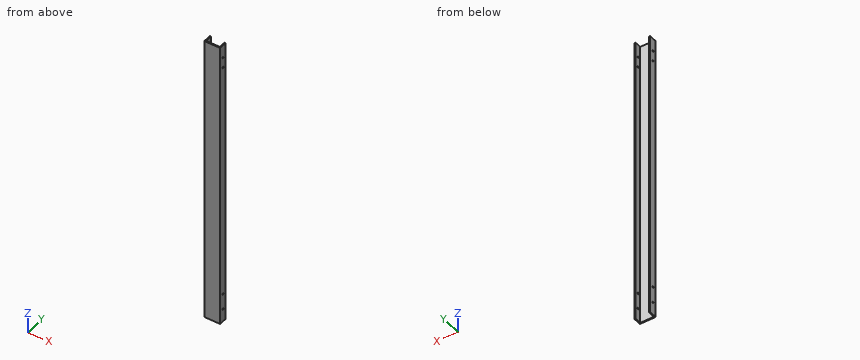
from build123d import *

# Parameters (mm, degrees)
EXTRUDE_1_DEPTH = 560.3
M4X0_7_1_D      = 3.3
M4X0_7_1_DEPTH  = 11.5
M4X0_7_1_TIP    = 0.991420021
M4X0_7_2_D      = 3.3
M4X0_7_2_DEPTH  = 11.5
M4X0_7_2_TIP    = 0.991420021
M4X0_7_4_D      = 3.3
M4X0_7_4_DEPTH  = 11.5
M4X0_7_4_TIP    = 0.991420021


with BuildPart() as part:
    # ｽｹｯﾁ1 → ﾎﾞｽ - 押し出し1 (new body)
    with BuildSketch(Plane.XY):
        Polygon((0, 0), (15, 0), (15, 15), (13, 15), (13, 2), (-13, 2), (-13, 15), (-15, 15), (-15, 0), align=None)
    extrude(amount=EXTRUDE_1_DEPTH)

    # M4x0.7 ねじ穴1
    with Locations(Plane(origin=(15, 7.5, 56), x_dir=(0, 0, 1), z_dir=(1, 0, 0))):
        with Locations((0, 0), (-31, 0)):
            Hole(M4X0_7_1_D / 2, depth=M4X0_7_1_DEPTH)
            with Locations((0, 0, -(M4X0_7_1_DEPTH + M4X0_7_1_TIP / 2))):  # 118° drill point
                Cone(0, M4X0_7_1_D / 2, M4X0_7_1_TIP, mode=Mode.SUBTRACT)

    # M4x0.7 ねじ穴2
    with Locations(Plane(origin=(15, 7.5, 535.3), x_dir=(0, 0, 1), z_dir=(1, 0, 0))):
        with Locations((0, 0), (-20, 0)):
            Hole(M4X0_7_2_D / 2, depth=M4X0_7_2_DEPTH)
            with Locations((0, 0, -(M4X0_7_2_DEPTH + M4X0_7_2_TIP / 2))):  # 118° drill point
                Cone(0, M4X0_7_2_D / 2, M4X0_7_2_TIP, mode=Mode.SUBTRACT)

    # M4x0.7 ねじ穴4
    with Locations(Plane(origin=(-15, 7.5, 56), x_dir=(0, 0, -1), z_dir=(-1, 0, 0))):
        with Locations((0, 0), (31, 0), (-459.3, 0), (-479.3, 0)):
            Hole(M4X0_7_4_D / 2, depth=M4X0_7_4_DEPTH)
            with Locations((0, 0, -(M4X0_7_4_DEPTH + M4X0_7_4_TIP / 2))):  # 118° drill point
                Cone(0, M4X0_7_4_D / 2, M4X0_7_4_TIP, mode=Mode.SUBTRACT)


solid = part.part
Check sheet for the modelled part. Datum: model origin and axes. Units: mm. Give positions to 0.01 mm unless a question says otherwise; leave off trailing zeros. Write each loop counter-clockwise with the first axis right and the second up, starting at its lowest first coordinate (ties: lowest second). Pieces come first, ordered by that corner, then holes. Notation, with made-up numbers: (17, 24) -> (68, 24) arc R14 ccw to (68, 31) -> close; hole circle Ø8 at (68.25, -34). An arc over 180 degrees is marked (long way). Use one line per item in the form item = value. Start each with the question number.
1. Section check B-B (x = -6). Record the cut outline in (y, z).
2. Thickness scan on line 1 along Z through (x, y) = (14.1, 7.5); line 2 along X through (y, z) = (5.5, 154.5); line 3 along Y through (x, z) = (-13.4, 56). Record the ranges inside material, lowest first. Write a range as from..to.
3. Section check A-A (z = 363.5). Record the cut outline in (x, y), and give its area (3 significant figures).
4. Go/stop test with flat-tipped pins: P1, Ø2.5, axis at y = 7.5, z = 56, coming from the -X side; P2, Ø1.5, axis at x = 10, z = 77.5, coming from the +Y side. Record where each tip stops, or that it passes through.
Conclusion:
q1.outline = (0, 0) -> (2, 0) -> (2, 560.3) -> (0, 560.3) -> close
q2.line_1 = 0..23.35, 26.65..54.35, 57.65..513.65, 516.95..533.65, 536.95..560.3
q2.line_2 = -15..-13, 13..15
q2.line_3 = 0..5.85, 9.15..15
q3.outline = (-15, 0) -> (15, 0) -> (15, 15) -> (13, 15) -> (13, 2) -> (-13, 2) -> (-13, 15) -> (-15, 15) -> close
q3.area = 112 mm²
q4.P1 = through
q4.P2 = 2
